Can you work these out from the model? Positions are in its coordinate system, mm. Face numbers are marked on the shaded views. A direction names the side the tool comes from. Give positions to 0.01 mm unless a question says otherwise; leave off trailing zeros. Order: outer loops, then holes, each group sorted by start corner. A loop starts at its lowest first (then second) coordinate and runs counter-clockwise, first axis right, second up. Notation, with made-up numbers: (65.5, 68.5) -> (121.5, 68.5) arc R19 ccw to (121.5, 84.5) -> close; hole circle Ø1 at (39.25, -14). An arc over 180 degrees is marked (long way). Answer as CSV lines item,"result".
```python
from build123d import *

# Parameters (mm, degrees)
F1_DEPTH = 6.35


with BuildPart() as f1:
    # F0 (on Front) → F1 (new body)
    with BuildSketch(Plane.XZ):
        with BuildLine():
            Line((0.498749, 15.24), (-2.041251, 15.24))
            ThreePointArc((-2.041251, 15.24), (-2.490083, 13.877276), (-2.54, 12.443408))
            ThreePointArc((-2.54, 12.443408), (-3.578003, 12.185561), (-4.59063, 11.841289))
            ThreePointArc((-4.59063, 11.841289), (-6.095514, 12.749414), (-7.819791, 13.090348))
            Line((-7.819791, 13.090348), (-9.956575, 11.71712))
            ThreePointArc((-9.956575, 11.71712), (-9.597413, 10.328067), (-8.864198, 9.094833))
            ThreePointArc((-8.864198, 9.094833), (-9.59802, 8.316731), (-10.263768, 7.479644))
            ThreePointArc((-10.263768, 7.479644), (-12.020726, 7.430005), (-13.655604, 6.784603))
            Line((-13.655604, 6.784603), (-14.710758, 4.474138))
            ThreePointArc((-14.710758, 4.474138), (-13.657632, 3.499769), (-12.374076, 2.858713))
            ThreePointArc((-12.374076, 2.858713), (-12.570732, 1.807398), (-12.678232, 0.743265))
            ThreePointArc((-12.678232, 0.743265), (-14.129443, -0.248377), (-15.155858, -1.675205))
            Line((-15.155858, -1.675205), (-14.794379, -4.189352))
            ThreePointArc((-14.794379, -4.189352), (-13.381649, -4.43968), (-11.955272, -4.285028))
            ThreePointArc((-11.955272, -4.285028), (-11.552326, -5.275771), (-11.067446, -6.229095))
            ThreePointArc((-11.067446, -6.229095), (-11.752161, -7.847902), (-11.844235, -9.603148))
            Line((-11.844235, -9.603148), (-10.180889, -11.522752))
            ThreePointArc((-10.180889, -11.522752), (-8.857087, -10.969562), (-7.740754, -10.068303))
            ThreePointArc((-7.740754, -10.068303), (-6.866138, -10.68392), (-5.942825, -11.223762))
            ThreePointArc((-5.942825, -11.223762), (-5.643651, -12.955773), (-4.772151, -14.482159))
            Line((-4.772151, -14.482159), (-2.335039, -15.19776))
            ThreePointArc((-2.335039, -15.19776), (-1.520463, -14.016686), (-1.068601, -12.654963))
            ThreePointArc((-1.068601, -12.654963), (0, -12.7), (1.068601, -12.654963))
            ThreePointArc((1.068601, -12.654963), (2.256678, -13.950278), (3.815058, -14.763187))
            Line((3.815058, -14.763187), (6.25217, -14.047586))
            ThreePointArc((6.25217, -14.047586), (6.298898, -12.613611), (5.942825, -11.223762))
            ThreePointArc((5.942825, -11.223762), (6.866138, -10.68392), (7.740754, -10.068303))
            ThreePointArc((7.740754, -10.068303), (9.440528, -10.515668), (11.191012, -10.357007))
            Line((11.191012, -10.357007), (12.854358, -8.437403))
            ThreePointArc((12.854358, -8.437403), (12.118403, -7.205804), (11.067446, -6.229095))
            ThreePointArc((11.067446, -6.229095), (11.552326, -5.275771), (11.955272, -4.285028))
            ThreePointArc((11.955272, -4.285028), (13.627077, -3.742408), (15.013899, -2.662551))
            Line((15.013899, -2.662551), (15.375379, -0.148405))
            ThreePointArc((15.375379, -0.148405), (14.090401, 0.489796), (12.678232, 0.743265))
            ThreePointArc((12.678232, 0.743265), (12.570732, 1.807398), (12.374076, 2.858713))
            ThreePointArc((12.374076, 2.858713), (13.487125, 4.21904), (14.06998, 5.877246))
            Line((14.06998, 5.877246), (13.014826, 8.187712))
            ThreePointArc((13.014826, 8.187712), (11.588796, 8.029888), (10.263768, 7.479644))
            ThreePointArc((10.263768, 7.479644), (9.59802, 8.316731), (8.864198, 9.094833))
            ThreePointArc((8.864198, 9.094833), (9.065106, 10.840973), (8.658941, 12.55106))
            Line((8.658941, 12.55106), (6.522157, 13.924287))
            ThreePointArc((6.522157, 13.924287), (5.40783, 13.020548), (4.59063, 11.841289))
            ThreePointArc((4.59063, 11.841289), (3.578003, 12.185561), (2.54, 12.443408))
            ThreePointArc((2.54, 12.443408), (1.76498, 14.020973), (0.498749, 15.24))
        make_face()
        with BuildLine():
            ThreePointArc((-1.524, -6.164408), (-3.914403, 4.999995), (6.35, 0))
            ThreePointArc((6.35, 0), (4.999995, -3.914403), (1.524, -6.164408))
            Line((1.524, -6.164408), (1.524, -8.89))
            Line((1.524, -8.89), (0, -8.89))
            Line((0, -8.89), (-1.524, -8.89))
            Line((-1.524, -8.89), (-1.524, -6.164408))
        make_face(mode=Mode.SUBTRACT)
    extrude(amount=F1_DEPTH)


solid = f1.part
```
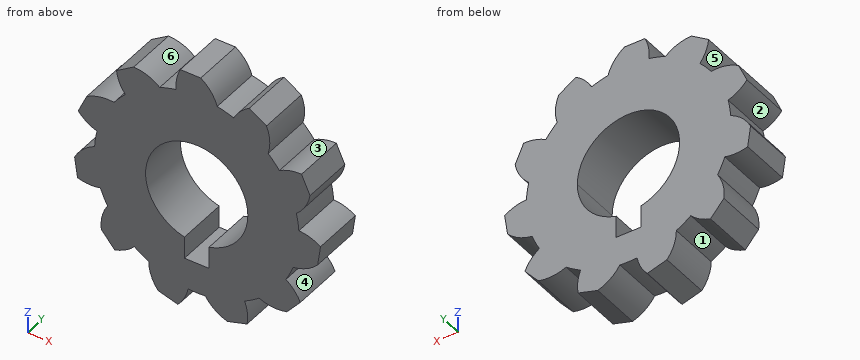
Item 1: For the marked faces 1, 2 and 3, which set-ups out of +Z, -Z, +X, -X, +Y, -Y let a thin tool reach every point of the face, with its end or its side?
Numbers:
face 1,"-Z, +Y, -Y"
face 2,"-X, +Y, -Y"
face 3,"+Z, +Y, -Y"
Item 2: Imagine slicing it at B-B, the plane x = 0. Please give me the cut outline in (y, z).
Numbers:
outline,"(-6.35, -12.7) -> (0, -12.7) -> (0, -8.89) -> (-6.35, -8.89) -> close; (-6.35, 6.35) -> (0, 6.35) -> (0, 15.24) -> (-6.35, 15.24) -> close"
Item 3: For pin 1 (2 mm diameter, centred on y = -2, z = -7.5, fed in from +X); pin 2 (0.8 mm diameter, centred on y = -4, z = -7, fed in from -X), each with a flat end and sliding along its axis, tell me the tip position at first contact or that it passes through.
Numbers:
pin 1,"stops at x = 12.85"
pin 2,"stops at x = -11.63"
Item 4: We'd pull the mould along X, two halves only. Please class the marked faces 4, 5 and 6: released by +X, released by -X, zero draft, split by the parting line, or undercut.
Numbers:
face 4,"released by +X"
face 5,"released by -X"
face 6,"undercut"
Item 5: Please list where these lines run through material, in increasing order: line 1 along X through (y, z) = (-0.25, 1); line 2 along X through (y, z) = (-4.75, -9); line 3 along Z through (x, y) = (-2, -2) (3 decimals).
Numbers:
line 1,"x = -12.66 to -6.27, 6.27 to 12.66"
line 2,"x = -11.88 to 12.37"
line 3,"z = -14.795 to -6.027, 6.027 to 15.24"
Item 6: Imagine slicing it at A-A, the plane z = 1.5. Please give me the cut outline in (x, y), then the cut area to 3 significant figures.
Numbers:
outline,"(-12.61, -6.35) -> (-6.17, -6.35) -> (-6.17, 0) -> (-12.61, 0) -> close; (6.17, -6.35) -> (12.61, -6.35) -> (12.61, 0) -> (6.17, 0) -> close"
area,"81.8 mm²"
